The listing builds one solid part. Answer for the finished solid, in the listing's coordinates (mm). Face numbers are marked on the shaded views. A direction names the side the tool comes from. Coordinates: 2 decimals unless noted, no trailing zeros. Write each loop counter-clockwise with the first axis right and the second up, starting at its lowest first coordinate (ties: lowest second). Pieces come first, ordered by that corner, then holes.
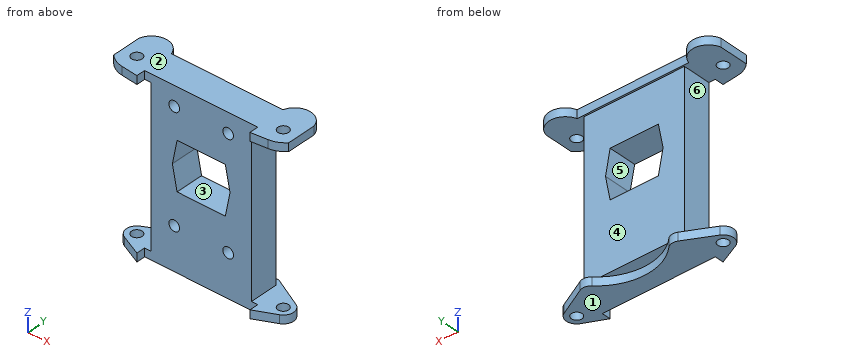
from build123d import *

# Parameters (mm, degrees)
SKETCH1_W           = 37.211
SKETCH1_H           = 57.658
BOSS_EXTRUDE1_DEPTH = 10.4394
BOSS_EXTRUDE2_DEPTH = 3.048
BOSS_EXTRUDE3_DEPTH = 3.048
SKETCH5_R           = 1.9685
CUT_EXTRUDE1_DEPTH  = 74.180460976
SKETCH6_R           = 1.9685
CUT_EXTRUDE2_DEPTH  = 5.08


with BuildPart() as part:
    # Sketch1 → Boss-Extrude1 (new body)
    with BuildSketch(Plane(origin=(0, 0, 0), x_dir=(1, 0, 0), z_dir=(0, 1, 0))):
        Rectangle(SKETCH1_W, SKETCH1_H)
        Polygon((-8.949851054, 4.0894), (8.949851054, 4.0894), (10.6807, -4.7498), (8.949851054, -13.589), (-8.949851054, -13.589), (-10.6807, -4.7498), align=None, mode=Mode.SUBTRACT)
    extrude(amount=BOSS_EXTRUDE1_DEPTH)

    # Sketch2 → Boss-Extrude2 (add)
    with BuildSketch(Plane.XY.offset(28.829)):
        with BuildLine():
            Line((-20.701, 11.049), (20.701, 11.049))
            ThreePointArc((20.701, 11.049), (26.723405801, 15.394332642), (32.4612, 10.679568052))
            Line((32.4612, 10.679568052), (32.4612, 0))
            ThreePointArc((32.4612, 0), (29.989172762, -1.802849379), (27.049629295, -2.651535867))
            Line((27.049629295, -2.651535867), (20.9677, -3.302))
            Line((20.9677, -3.302), (20.9677, 0))
            Line((20.9677, 0), (-20.9677, 0))
            Line((-20.9677, 0), (-20.9677, -3.302))
            Line((-20.9677, -3.302), (-27.049629295, -2.651535867))
            ThreePointArc((-27.049629295, -2.651535867), (-29.989172762, -1.802849379), (-32.4612, 0))
            Line((-32.4612, 0), (-32.4612, 10.679568052))
            ThreePointArc((-32.4612, 10.679568052), (-26.723405801, 15.394332642), (-20.701, 11.049))
        make_face()
    extrude(amount=BOSS_EXTRUDE2_DEPTH)

    # Sketch3 → Boss-Extrude3 (add)
    with BuildSketch(Plane(origin=(0, 0, -28.829), x_dir=(-1, 0, 0), z_dir=(0, 0, -1))):
        with BuildLine():
            Line((18.175030658, 12.62989205), (28.898610874, 7.159054501))
            ThreePointArc((28.898610874, 7.159054501), (30.974624731, 3.696565568), (28.769674487, 0.314723233))
            Line((28.769674487, 0.314723233), (20.9677, -3.302))
            Line((20.9677, -3.302), (20.9677, 0))
            Line((20.9677, 0), (0, 0))
            Line((0, 0), (-20.9677, 0))
            Line((-20.9677, 0), (-20.9677, -3.302))
            Line((-20.9677, -3.302), (-28.769674487, 0.314723233))
            ThreePointArc((-28.769674487, 0.314723233), (-30.974624731, 3.696565568), (-28.898610874, 7.159054501))
            Line((-28.898610874, 7.159054501), (-18.175030658, 12.62989205))
            ThreePointArc((-18.175030658, 12.62989205), (-16.096634608, 12.965404658), (-14.213319827, 12.024434793))
            ThreePointArc((-14.213319827, 12.024434793), (0, 6.223), (14.213319827, 12.024434793))
            ThreePointArc((14.213319827, 12.024434793), (16.096634608, 12.965404658), (18.175030658, 12.62989205))
        make_face()
    extrude(amount=BOSS_EXTRUDE3_DEPTH)

    # Sketch5 → Cut-Extrude1 (cut, through all)
    with BuildSketch(Plane(origin=(0, 0, -31.877), x_dir=(-1, 0, 0), z_dir=(0, 0, -1))):
        with Locations((-27.16873413, 3.768262533)):
            Circle(SKETCH5_R)
        with Locations((27.16873413, 3.768262533)):
            Circle(SKETCH5_R)
    extrude(amount=-CUT_EXTRUDE1_DEPTH, mode=Mode.SUBTRACT)

    # Sketch6 → Cut-Extrude2 (cut)
    with BuildSketch(Plane.XZ):
        with Locations(Location((-10.0076, 24.6507, 0), (0, 0, 270))):
            Circle(SKETCH6_R)
        with Locations(Location((10.0076, 24.6507, 0), (0, 0, 270))):
            Circle(SKETCH6_R)
        with Locations(Location((-10.0076, -16.1417, 0), (0, 0, 270))):
            Circle(SKETCH6_R)
        with Locations(Location((10.0076, -16.1417, 0), (0, 0, 270))):
            Circle(SKETCH6_R)
    extrude(amount=-CUT_EXTRUDE2_DEPTH, mode=Mode.SUBTRACT)


solid = part.part
Q1. Find the intervals of material crossed by probe 1 along Z at (x, y) = (-4.5, 3); probe 2 along Z at (x, y) = (21, 8.5); probe 3 along X at (y, z) = (4.5, -20.5), in increasing order.
Answers below:
probe 1: z = -31.88 to -4.09, 13.59 to 31.88
probe 2: z = -31.88 to -28.83, 28.83 to 31.88
probe 3: x = -18.61 to 18.61
Q2. The part is cut by section A-A, the plane x = 0. Write down the section's boundary in (y, z), then the cut area to 3 significant figures.
Answers below:
outline: (0, -31.88) - (6.22, -31.88) - (6.22, -28.83) - (10.44, -28.83) - (10.44, -4.09) - (0, -4.09) - close; (0, 13.59) - (10.44, 13.59) - (10.44, 28.83) - (11.05, 28.83) - (11.05, 31.88) - (0, 31.88) - close
area: 470 mm2
Q3. Which of the six approach directions +Z, -Z, +X, -X, +Y, -Y give full straight-line access (tool end or side, diameter ignored) to the marked faces 4, 5 and 6?
Answers below:
face 4: +X, -X, +Y
face 5: +Y, -Y
face 6: -X, +Y, -Y
Q4. The part is cut by section D-D, the plane y = 2.75. State how many separate pieces and enclosed holes the cut face has, then the cut area to 3 significant figures.
Answers below:
separate pieces: 5
enclosed holes: 5
area: 2,090 mm2
Q5. The part is cut by section B-B, the plane z = 2.5. Write down the section's boundary in (x, y), then the cut area to 3 significant figures.
Answers below:
outline: (-18.61, 0) - (-10.24, 0) - (-10.24, 10.44) - (-18.61, 10.44) - close; (10.24, 0) - (18.61, 0) - (18.61, 10.44) - (10.24, 10.44) - close
area: 175 mm2
Q6. The part is cut by section C-C, the plane x = 24. Write down the section's boundary in (y, z).
Answers below:
outline: (-2.98, 28.83) - (14.85, 28.83) - (14.85, 31.88) - (-2.98, 31.88) - close; (-1.9, -31.88) - (9.66, -31.88) - (9.66, -28.83) - (-1.9, -28.83) - close
Q7. Determine the mould class of the marked faces 1, 2 and 3 for opening direction Z: released by +Z, released by -Z, zero draft, split by the parting line, or undercut.
Answers below:
face 1: released by -Z
face 2: released by +Z
face 3: undercut
Q8. Given pin 1 (3 mm diameter, centred on x = -10.5, z = 24, fed in from -Y); pin 2 (3.5 mm diameter, centred on y = -2.5, z = 30, fed in from +X); pin 3 (5 mm diameter, centred on y = 5, z = 19, fed in from -X), each flat-ended and moving along its own axis, determine where each tip first touches the part or whether it passes through.
Answers below:
pin 1: stops at y = 0
pin 2: stops at x = 31.64
pin 3: stops at x = -18.61
